Could you check a few things on this model? Use its own coordinates, in mm. A direction names the side the tool comes from. Give positions to 0.01 mm unless a question says otherwise; leave off trailing zeros. Order: outer loops, then holes, each group sorted by start corner. A loop starts at its lowest first (then second) coordinate and runs counter-clockwise, first axis right, second up. Notation, with made-up numbers: (76.5, 59.5) - (92.5, 59.5) arc R10 cw to (92.5, 67.5) - close; hole circle Ø5 at (68, 76.5). An arc over 180 degrees is marked (long way). Put each result on its own line as item: value.
from build123d import *

# Parameters (mm, degrees)
SKETCH1_W           = 56.2
SKETCH1_H           = 26.75
SKETCH1_R           = 2.5
SKETCH1_W_2         = 40.2
SKETCH1_H_2         = 20.4
BOSS_EXTRUDE1_DEPTH = 3.175
SKETCH2_W           = 56.2
SKETCH2_H           = 3.175
BOSS_EXTRUDE2_DEPTH = 28
SKETCH3_R           = 1.25
CUT_EXTRUDE1_DEPTH  = 3.175


with BuildPart() as part:
    # Sketch1 → Boss-Extrude1 (new body)
    with BuildSketch(Plane(origin=(0, 0, 0), x_dir=(1, 0, 0), z_dir=(0, 1, 0))):
        Rectangle(SKETCH1_W, SKETCH1_H)
        with Locations(Location((24.8, 5, 0), (0, 0, 270))):
            Circle(SKETCH1_R, mode=Mode.SUBTRACT)
        with Locations(Location((24.8, -5, 0), (0, 0, 270))):
            Circle(SKETCH1_R, mode=Mode.SUBTRACT)
        with Locations(Location((-24.8, -5, 0), (0, 0, 90))):
            Circle(SKETCH1_R, mode=Mode.SUBTRACT)
        with Locations(Location((-24.8, 5, 0), (0, 0, 90))):
            Circle(SKETCH1_R, mode=Mode.SUBTRACT)
        Rectangle(SKETCH1_W_2, SKETCH1_H_2, mode=Mode.SUBTRACT)
    extrude(amount=BOSS_EXTRUDE1_DEPTH)

    # Sketch2 → Boss-Extrude2 (add)
    with BuildSketch(Plane(origin=(0, 0, 0), x_dir=(-1, 0, 0), z_dir=(0, -1, 0))):
        with Locations((0, -11.7875)):
            Rectangle(SKETCH2_W, SKETCH2_H)
    extrude(amount=BOSS_EXTRUDE2_DEPTH)

    # Sketch3 → Cut-Extrude1 (cut)
    with BuildSketch(Plane.XY.offset(13.375)):
        with Locations((-9.75, -5.953329294)):
            Circle(SKETCH3_R)
        with Locations((-13.75, -5.953329294)):
            Circle(SKETCH3_R)
    extrude(amount=-CUT_EXTRUDE1_DEPTH, mode=Mode.SUBTRACT)


solid = part.part
1) Suppose I cut it at D-D, the plane y = -18. List the corners of the cut face in (x, z) for me (3 decimals), and give its area (3 significant figures).
Filled in:
outline: (-28.1, 10.2) - (28.1, 10.2) - (28.1, 13.375) - (-28.1, 13.375) - close
area: 178 mm^2
2) We'd pull the mould along Y, two halves only. Please class faces 4 (the flat face through (0, 3.175, 11)), 5 (the flat face through (0, -12, 10.2)), 6 (the cylindrical face through (-11, -6, 12)): pulls with the +Y half, pulls with the -Y half, needs draft (parallel to the pull), parting line crosses it, or undercut.
Filled in:
face 4: pulls with the +Y half
face 5: needs draft
face 6: undercut
3) Suppose I cut it at B-B, the plane x = 24.8. List the corners of the cut face in (y, z) for me (3 decimals), and give its area (3 significant figures).
Filled in:
outline: (-28, 10.2) - (0, 10.2) - (0, 7.5) - (3.175, 7.5) - (3.175, 13.375) - (-28, 13.375) - close; (0, -13.375) - (3.175, -13.375) - (3.175, -7.5) - (0, -7.5) - close; (0, -2.5) - (3.175, -2.5) - (3.175, 2.5) - (0, 2.5) - close
area: 142 mm^2
4) I'm going to push a flat-ended pin straight in: pin 1 (4 mm diameter, centred on x = -16.5, y = -15.5, fed in from -Z). Where does the tip first touch, or does it pass through?
Filled in:
pin 1: stops at z = 10.2
5) Suppose I cut it at C-C, the plane z = 1.25. List the corners of the cut face in (x, y) for me (3 decimals), and give its area (3 significant figures).
Filled in:
outline: (-28.1, 0) - (-20.1, 0) - (-20.1, 3.175) - (-28.1, 3.175) - close; (20.1, 0) - (28.1, 0) - (28.1, 3.175) - (20.1, 3.175) - close
area: 50.8 mm^2
6) If I drill on line 1 (X direction, y = 1.15, z = 5); line 2 (Y direction, x = -13.75, z = 11.9) (3 decimals); line 3 (Z direction, x = 24, y = 1) (3 decimals), over which ranges is the centre line in solid material (lowest first)? Write a range as [from, to].
Filled in:
line 1: x = [-28.1, -27.3], [-22.3, -20.1], [20.1, 22.3], [27.3, 28.1]
line 2: y = [-28, -7.203], [-4.703, 3.175]
line 3: z = [-13.375, -7.369], [-2.631, 2.631], [7.369, 13.375]
7) Which directions (+Z, -Z, +X, -X, +Y, -Y) give clear straight access to the entire face, cutting with the end or side of a thin tool? Please do faces 1 (the flat face through (-20.1, 2, 0)), 2 (the flat face through (2, 0, -10.4)), 3 (the cylindrical face through (-14.67, -5.11, 11.81)).
Filled in:
face 1: +Y, -Y
face 2: -Z, +X, -X, -Y
face 3: +Z, -Z
8) Suppose I cut it at A-A, the plane z = 5. List the corners of the cut face in (x, y) for me (3 decimals), and give its area (4 significant figures).
Filled in:
outline: (-28.1, 0) - (-27.3, 0) - (-27.3, 3.175) - (-28.1, 3.175) - close; (-22.3, 0) - (-20.1, 0) - (-20.1, 3.175) - (-22.3, 3.175) - close; (20.1, 0) - (22.3, 0) - (22.3, 3.175) - (20.1, 3.175) - close; (27.3, 0) - (28.1, 0) - (28.1, 3.175) - (27.3, 3.175) - close
area: 19.05 mm^2
